Study the drawing (mm; zero at the part's minimum x, y, z) and answer. A direction names the side the tool comes from. Round coordinates to 2 decimals unless told otherwise and drop trailing zeros. Write each loop counter-clockwise with the first axis right and the second up, starting at its lowest first coordinate (ties: lowest second). Pieces come first, ordered by that corner, then holes. Notation, with made-up numbers: (-20, 57) -> (23, 57) arc R14 ccw to (23, 78) -> close; hole circle Ø6 at (28, 16). An arc over 180 degrees is marked (long way). Return JSON: item names as keys, results as strings.
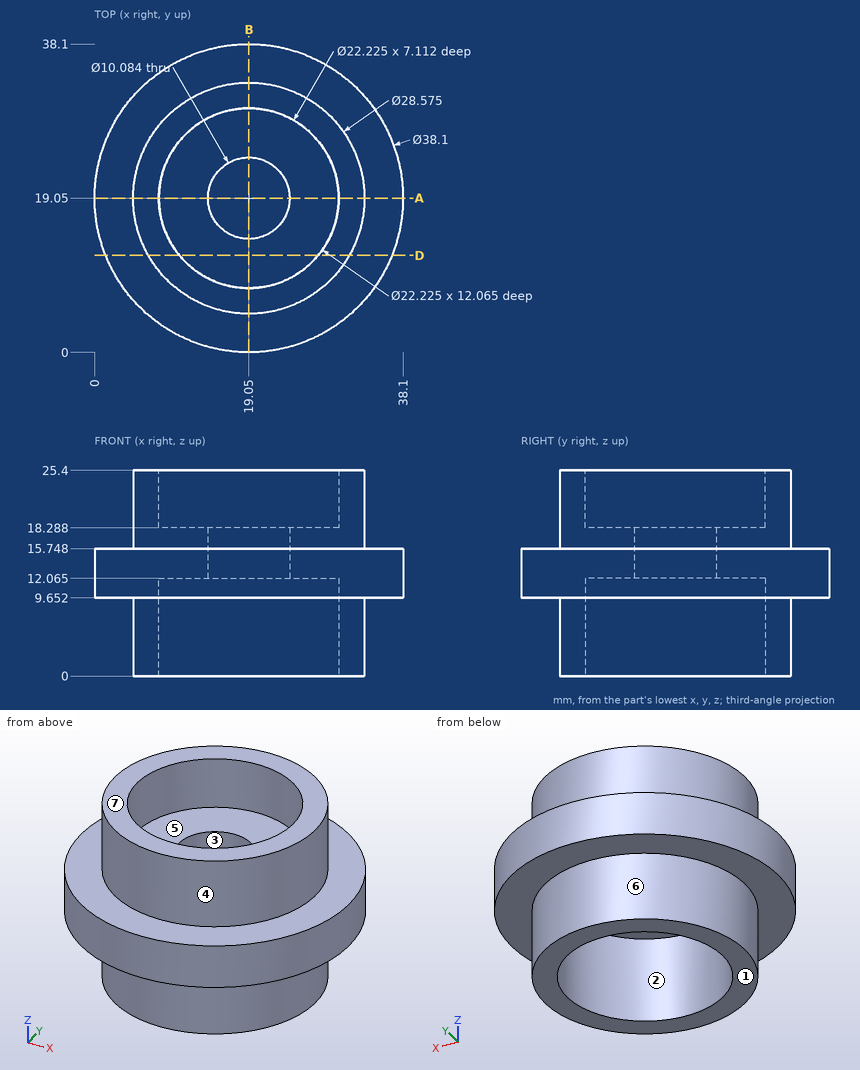
Item 1: A tool of negligible diameter and unlimited length cuts with its end or side. For the marked faces 5, 6 and 7, from which of +Z, -Z, +X, -X, +Y, -Y can it reach the whole face along a straight path? Write none if from no direction.
Worked answers:
{"face 5": "+Z", "face 6": "-Z", "face 7": "+Z, +X, -X, +Y, -Y"}
Item 2: Section D-D (y = 12) is taken. Give the vertices of the cut face in (x, z) (1 decimal), then the cut area to 3 significant figures.
Worked answers:
{"outline": "(1.4, 9.7) -> (6.6, 9.7) -> (6.6, 0) -> (10.5, 0) -> (10.5, 12.1) -> (27.6, 12.1) -> (27.6, 0) -> (31.5, 0) -> (31.5, 9.7) -> (36.7, 9.7) -> (36.7, 15.7) -> (31.5, 15.7) -> (31.5, 25.4) -> (27.6, 25.4) -> (27.6, 18.3) -> (10.5, 18.3) -> (10.5, 25.4) -> (6.6, 25.4) -> (6.6, 15.7) -> (1.4, 15.7) -> close", "area": "366 mm2"}
Item 3: Straight lines are drawn through the part: L1, parallel to Z at x = 17, y = 35; L2, parallel to Y at x = 12, z = 4.75; L3, parallel to Y at x = 14.5, z = 7.75. For each, find the intervals that lie inside material, in ascending order. Write a range as [from, to].
Worked answers:
{"L1": "z = [9.65, 15.75]", "L2": "y = [6.62, 10.46], [27.64, 31.48]", "L3": "y = [5.51, 8.91], [29.19, 32.59]"}
Item 4: Section A-A (y = 19.05) is taken. Give the vertices of the cut face in (x, z) (1 decimal).
Worked answers:
{"outline": "(0, 9.7) -> (4.8, 9.7) -> (4.8, 0) -> (7.9, 0) -> (7.9, 12.1) -> (14, 12.1) -> (14, 18.3) -> (7.9, 18.3) -> (7.9, 25.4) -> (4.8, 25.4) -> (4.8, 15.7) -> (0, 15.7) -> close; (24.1, 12.1) -> (30.2, 12.1) -> (30.2, 0) -> (33.3, 0) -> (33.3, 9.7) -> (38.1, 9.7) -> (38.1, 15.7) -> (33.3, 15.7) -> (33.3, 25.4) -> (30.2, 25.4) -> (30.2, 18.3) -> (24.1, 18.3) -> close"}
Item 5: Flat-ended cylindrical pins translate along their axes: pin 1 (18 mm diameter, centred on x = 20.5, y = 18.5, fed in from +Z); pin 2 (6.5 mm diameter, centred on x = 14.5, y = 19.5, fed in from -Z) (3 decimals); pin 3 (11.5 mm diameter, centred on x = 12.5, y = 19, fed in from +Z); pin 4 (6 mm diameter, centred on y = 7, z = 21, fed in from +X). Find the tip coordinate at first contact, or state that the pin passes through.
Worked answers:
{"pin 1": "stops at z = 18.29", "pin 2": "stops at z = 12.065", "pin 3": "stops at z = 25.4", "pin 4": "stops at x = 30.11"}
Item 6: For a pull along X with two mould halves and no side action, classify the marked faces 1, 2, 3 and 4 as released by +X, released by -X, zero draft, split by the parting line, or undercut.
Worked answers:
{"face 1": "zero draft", "face 2": "undercut", "face 3": "undercut", "face 4": "split by the parting line"}
